Part model, mm, in its own coordinate system. A direction names the side the tool comes from. Give positions to 0.01 mm unless a question says otherwise; leave off trailing zeros. Write each loop counter-clockwise with the first axis right and the second up, starting at its lowest first coordinate (ties: lowest second). Pieces come first, ordered by that corner, then holes. Notation, with made-up numbers: (26, -8) - (48, -8) arc R14 ccw to (48, -2) - close; hole circle Ø1 at (65.25, -24.5). An arc over 180 degrees is marked (long way). Answer in a Markdown table with one row per item. Add a question column.
1. Drop flat-ended pins along their axis: pin 1 Ø3 at (y, z) = (-2, 43.5) entering from -X; pin 2 Ø1.5 at (y, z) = (-0.5, 26.5) entering from +X; pin 3 Ø1.5 at (x, z) = (2.5, 55) entering from -Y. Give the stop position or say it passes through.
2. Band-saw the part on A-A on x = -0.6. Write the cut outline in (y, z).
3. Which spindle directions (+Z, -Z, +X, -X, +Y, -Y) get a long thin tool onto all of the face, cutting with end or side? Do faces 1 (the flat face through (-2, 2, 72)), 2 (the cylindrical face through (0.54, -2.44, -29.52)), 3 (the cylindrical face through (-3, 0, 23)). Say none if no direction does.
4. Band-saw the part on C-C on z = 13. Write the cut outline in (x, y), plus the area to 3 significant figures.
5. Band-saw the part on B-B on y = -1.2. Write the cut outline in (x, z).
6. Probe line 1 along X through (y, z) = (0.15, 21); line 2 along Z through (x, y) = (-2.2, 1.3). List the from-to ranges inside material, lowest first.
```python
from build123d import *

# Parameters (mm, degrees)
SKETCH2_R                = 3
BOSS_EXTRUDE1_DEPTH      = 75
BOSS_EXTRUDE1_DEPTH_BACK = 75
CHAMFER1_SIZE            = 0.12
SKETCH4_R                = 3
CUT_EXTRUDE1_DEPTH       = 44
SKETCH5_OUTSIDE_W        = 29.268
SKETCH5_OUTSIDE_H        = 29.268
SKETCH5_OUTSIDE_R        = 2.5
CUT_EXTRUDE2_DEPTH       = 3
SKETCH6_OUTSIDE_W        = 29.268
SKETCH6_OUTSIDE_H        = 29.268
SKETCH6_OUTSIDE_R        = 2.5
CUT_EXTRUDE3_DEPTH       = 3


with BuildPart() as part:
    # Sketch2 → Boss-Extrude1 (new body, two sides)
    with BuildSketch(Plane.XY) as boss_extrude1_sk:
        Circle(SKETCH2_R)
    extrude(amount=BOSS_EXTRUDE1_DEPTH)
    extrude(boss_extrude1_sk.sketch, amount=-BOSS_EXTRUDE1_DEPTH_BACK)

    # Chamfer1
    chamfer1_edges = [part.edges().sort_by_distance(p)[0] for p in [
        (-3, 0, -75),
        (-3, 0, 75),
    ]]
    chamfer(chamfer1_edges, length=CHAMFER1_SIZE)

    # Sketch4 → Cut-Extrude1 (cut)
    with BuildSketch(Plane(origin=(0, 0, -75), x_dir=(-1, 0, 0), z_dir=(0, 0, -1))):
        Circle(SKETCH4_R)
    extrude(amount=-CUT_EXTRUDE1_DEPTH, mode=Mode.SUBTRACT)

    # Sketch5 outside → Cut-Extrude2 (cut)
    with BuildSketch(Plane(origin=(0, 0, -31), x_dir=(-1, 0, 0), z_dir=(0, 0, -1))):
        Rectangle(SKETCH5_OUTSIDE_W, SKETCH5_OUTSIDE_H)
        Circle(SKETCH5_OUTSIDE_R, mode=Mode.SUBTRACT)
    extrude(amount=-CUT_EXTRUDE2_DEPTH, mode=Mode.SUBTRACT)

    # Sketch6 outside → Cut-Extrude3 (cut)
    with BuildSketch(Plane.XY.offset(75)):
        Rectangle(SKETCH6_OUTSIDE_W, SKETCH6_OUTSIDE_H)
        Circle(SKETCH6_OUTSIDE_R, mode=Mode.SUBTRACT)
    extrude(amount=-CUT_EXTRUDE3_DEPTH, mode=Mode.SUBTRACT)


solid = part.part
```
Values:
| question | item | result |
|---|---|---|
| 1 | pin 1 | stops at x = -2.96 |
| 1 | pin 2 | stops at x = 3 |
| 1 | pin 3 | stops at y = -2.44 |
| 2 | outline | (-2.94, -28) - (-2.43, -28) - (-2.43, -31) - (2.43, -31) - (2.43, -28) - (2.94, -28) - (2.94, 72) - (2.43, 72) - (2.43, 75) - (-2.43, 75) - (-2.43, 72) - (-2.94, 72) - close |
| 3 | face 1 | +Z |
| 3 | face 2 | -Z |
| 3 | face 3 | +Z, -Z |
| 4 | outline | circle Ø6 at (0, 0) |
| 4 | area | 28.3 mm² |
| 5 | outline | (-2.75, -28) - (-2.19, -28) - (-2.19, -31) - (2.19, -31) - (2.19, -28) - (2.75, -28) - (2.75, 72) - (2.19, 72) - (2.19, 75) - (-2.19, 75) - (-2.19, 72) - (-2.75, 72) - close |
| 6 | line 1 | x = -3 to 3 |
| 6 | line 2 | z = -28 to 72 |
